Autodesk Inventor part; units mm, degrees
ref_plane "YZ Plane" through (0, 0, 0) normal (1, 0, 0) x (0, 1, 0)
ref_plane "XZ Plane" through (0, 0, 0) normal (0, 1, 0) x (-1, 0, 0)
ref_plane "XY Plane" through (0, 0, 0) normal (0, 0, 1) x (1, 0, 0)
sketch "Boceto1" plane through (0, 0, 0) normal (0, 1, 0) x (-1, 0, 0)
  arc A0 (81.875, -14.8824) -> (81.875, 14.8824) centre (80, 0) ccw
  line L0 (81.875, -14.8824) -> (3.125, -24.8039)
  line L1 (3.125, 24.8039) -> (81.875, 14.8824)
  line L2 (0, -32.0701) -> (0, 49.2426) construction
  arc A1 (-81.875, 14.8824) -> (-81.875, -14.8824) centre (-80, 0) ccw
  line L3 (-81.875, -14.8824) -> (-3.125, -24.8039)
  line L4 (-3.125, 24.8039) -> (-81.875, 14.8824)
  arc A2 (3.125, 24.8039) -> (-3.125, 24.8039) centre (0, 0) ccw
  arc A3 (-3.125, -24.8039) -> (3.125, -24.8039) centre (0, 0) ccw
  dimension "d1" = 30
  dimension "d2" = 80
extrude "Extrusión1" add sketch "Boceto1" along normal blind 25 draft 30 and the other way blind 10
sketch "Boceto2" plane through (0, -10, 0) normal (0, -1, 0) x (1, 0, 0)
  arc A0 (81.875, -14.8824) -> (81.875, 14.8824) centre (80, 0) ccw
  line L0 (81.875, 14.8824) -> (3.125, 24.8039)
  arc A1 (3.125, 24.8039) -> (-3.125, 24.8039) centre (0, 0) ccw
  line L1 (-3.125, 24.8039) -> (-81.875, 14.8824)
  arc A2 (-81.875, 14.8824) -> (-81.875, -14.8824) centre (-80, 0) ccw
  line L2 (-81.875, -14.8824) -> (-3.125, -24.8039)
  arc A3 (-3.125, -24.8039) -> (3.125, -24.8039) centre (0, 0) ccw
  line L3 (3.125, -24.8039) -> (81.875, -14.8824)
  circle A4 centre (0, 0) radius 17.1981
  circle A5 centre (-80, 0) radius 7.3963
  circle A6 centre (80, 0) radius 8.3739
extrude "Extrusión2" cut sketch "Boceto2" against normal through all contours A4 | A5 | A6
chamfer "Chaflán1" distance 2 angle 45 1 edges at (-87.3963, -10, 0)
chamfer "Chaflán2" distance 2 angle 45 1 edges at (-17.1981, -10, 0)
chamfer "Chaflán3" distance 2 angle 45 1 edges at (71.6261, -10, 0)
fillet "Empalme1" radius 1 8 edges at (0, -10, -25) (42.5, -10, -19.8431) (95, -10, 0) (42.5, -10, 19.8431) (0, -10, 25) (-42.5, -10, 19.8431) (-95, -10, 0) (-42.5, -10, -19.8431)
equation "\"Radio_pliegue\" = Grosor"
equation "\"Anchura_desahogo_plegado\" = Grosor"
equation "\"Profundidad_desahogo_plegado\" = 0.5 * Grosor"
equation "\"Tamaño_destalonado\" = 4 * Grosor"
equation "\"Remanente_mínimo\" = 2 * Grosor"
equation "\"Radiodetransición\" = Radio_pliegue"
equation "\"Tamaño_de_radio_de_Jacobi\" = Radio_pliegue"
equation "\"TamañoSeparación\" = Grosor"
properties part number "Practica4" material "Aluminio 6061-AHC"
Geometry: final body of the model. Coordinates: model frame, mm. A direction names the side the tool comes from. Give positions to 0.01 mm unless a question says otherwise; leave off trailing zeros. Write each loop counter-clockwise with the first axis right and the second up, starting at its lowest first coordinate (ties: lowest second). Pieces come first, ordered by that corner, then holes.
(1) Cut plane A-A, the plane x = 0. Return loops of the section in (y, z).
(2) First-contact query: P1, Ø2, axis at x = 18.5, y = 15.5, coming from the -Z side; P2, Ø2, axis at x = -73.5, y = 12.5, coming from the +Z side; P3, Ø1, axis at x = -19.5, y = 20, coming from the +Z side. Flat tips, straight axial feed; report the tip coordinate or a pass-through.
(3) Cut plane B-B, the plane z = 0. Return loops of the section in (x, y), then the cut area to 3 significant figures.
(4) Ray query, line 1 (Z direction, x = -80, y = 7); line 2 (X direction, y = 23, z = -1); line 3 (X direction, y = -6.5, z = -3). Return the intervals inside material, ascending.
(5) Cut plane C-C, the plane y = 9.5. Return loops of the section in (x, z), then the cut area to 3 significant figures.
(6) Access query for faces 1 (the cylindrical face through (0, -4, -25)), 2 (the flat face through (-41.949, -4.437, 19.913)), 3 (the cylindrical face through (95, -4, 0)). Directions: +Z, -Z, +X, -X, +Y, -Y. A direction counts if a zero-diameter tool reaches every point of the face in a straight line with its end or side. Return the directions, or none.
Values follow:
1. outline: (-10, -24) arc R1 ccw to (-9, -25) - (0, -25) - (25, -39.43) - (25, -17.2) - (-8, -17.2) - (-10, -19.2) - close; (-10, 19.2) - (-8, 17.2) - (25, 17.2) - (25, 39.43) - (0, 25) - (-9, 25) arc R1 ccw to (-10, 24) - close
2. P1: stops at z = -32.48
2. P2: stops at z = 23.81
2. P3: stops at z = 34.68
3. outline: (-109.43, 25) - (-95, 0) - (-95, -9) arc R1 ccw to (-94, -10) - (-89.4, -10) - (-87.4, -8) - (-87.4, 25) - close; (-72.6, -8) - (-70.6, -10) - (-19.2, -10) - (-17.2, -8) - (-17.2, 25) - (-72.6, 25) - close; (17.2, -8) - (19.2, -10) - (69.63, -10) - (71.63, -8) - (71.63, 25) - (17.2, 25) - close; (88.37, -8) - (90.37, -10) - (94, -10) arc R1 ccw to (95, -9) - (95, 0) - (109.43, 25) - (88.37, 25) - close
3. area: 4,690 mm2
4. line 1: z = -19.19 to -7.4, 7.4 to 19.19
4. line 2: x = -108.26 to -87.33, -72.67 to -17.17, 17.17 to 71.69, 88.31 to 108.26
4. line 3: x = -94.7 to -86.76, -73.24 to -16.93, 16.93 to 72.18, 87.82 to 94.7
5. outline: (-82.56, -20.32) - (-3.81, -30.25) arc R30.48 ccw to (3.81, -30.25) - (82.56, -20.32) arc R20.48 ccw to (82.56, 20.32) - (3.81, 30.25) arc R30.48 ccw to (-3.81, 30.25) - (-82.56, 20.32) arc R20.48 ccw to start; hole circle Ø14.79 at (-80, 0); hole circle Ø34.4 at (0, 0); hole circle Ø16.75 at (80, 0)
5. area: 8,220 mm2
6. face 1: -Z, -Y
6. face 2: +Z, -X, -Y
6. face 3: +X, -Y
